```python
from build123d import *

# Parameters (mm, degrees)
SKETCH1_R           = 16.5
BOSS_EXTRUDE1_DEPTH = 0.44
SKETCH2_R           = 0.85
SKETCH2_W           = 7
SKETCH2_H           = 1.75
CUT_EXTRUDE1_DEPTH  = 0.44


with BuildPart() as part:
    # Sketch1 → Boss-Extrude1 (new body)
    with BuildSketch(Plane(origin=(0, 0, 0), x_dir=(1, 0, 0), z_dir=(0, 1, 0))):
        Circle(SKETCH1_R)
    extrude(amount=BOSS_EXTRUDE1_DEPTH)

    # Sketch2 → Cut-Extrude1 (cut)
    with BuildSketch(Plane(origin=(0, 0.44, 0), x_dir=(1, 0, 0), z_dir=(0, 1, 0))):
        Circle(SKETCH2_R)
        with Locations((6.95, 0)):
            Rectangle(SKETCH2_W, SKETCH2_H)
    extrude(amount=-CUT_EXTRUDE1_DEPTH, mode=Mode.SUBTRACT)


solid = part.part
```
Source: CAD feature listing. Evaluate the final solid. Frame: model axes, mm. Coordinates: 2 decimals unless noted, no trailing zeros. Write each loop counter-clockwise with the first axis right and the second up, starting at its lowest first coordinate (ties: lowest second). Pieces come first, ordered by that corner, then holes. Notation, with made-up numbers: (1.5, 0) -> (37.5, 0) arc R26 cw to (37.5, 17) -> close; hole circle Ø6 at (-11.75, -4.5). An arc over 180 degrees is marked (long way). Return JSON: item names as keys, results as strings. Group by question number.
1) Section query A-A, the plane z = 0. Return loops of the section in (x, y), plus the area to 3 significant figures.
2) Mould query, pull axis X, two halves, no side actions, for faces 1 (the face through (15.24, 0.22, 6.32)), 2 (the face through (0, 0.44, 3)), 3 (the face through (-0.18, 0.22, 0.83)). Classes: +X half, -X half, draft (parallel to the pull), parting line (faces both ways), or undercut.
3) Section query C-C, the plane y = 0.35. Return loops of the section in (x, z) (3 decimals), plus the area to 3 significant figures.
4) Section query B-B, the plane x = 0. Return loops of the section in (y, z), plus the area to 3 significant figures.
5) Ray query, line 1 along X through (y, z) = (0.25, 0); line 2 along Z through (x, y) = (0, 0.1); line 3 along X through (y, z) = (0.3, 6). Return the intervals inside material, ascending.
6) Section query D-D, the plane x = 14.5. Return loops of the section in (y, z), plus the area to 3 significant figures.
From the geometry:
{
 "1": {"outline": "(-16.5, 0) -> (-0.85, 0) -> (-0.85, 0.44) -> (-16.5, 0.44) -> close; (0.85, 0) -> (3.45, 0) -> (3.45, 0.44) -> (0.85, 0.44) -> close; (10.45, 0) -> (16.5, 0) -> (16.5, 0.44) -> (10.45, 0.44) -> close", "area": "10.7 mm²"},
 "2": {"face 1": "parting line", "face 2": "draft", "face 3": "undercut"},
 "3": {"outline": "circle Ø33 at (0, 0); hole circle Ø1.7 at (0, 0); hole (3.45, -0.875) -> (10.45, -0.875) -> (10.45, 0.875) -> (3.45, 0.875) -> close", "area": "841 mm²"},
 "4": {"outline": "(0, -16.5) -> (0.44, -16.5) -> (0.44, -0.85) -> (0, -0.85) -> close; (0, 0.85) -> (0.44, 0.85) -> (0.44, 16.5) -> (0, 16.5) -> close", "area": "13.8 mm²"},
 "5": {"line 1": "-16.5 to -0.85, 0.85 to 3.45, 10.45 to 16.5", "line 2": "-16.5 to -0.85, 0.85 to 16.5", "line 3": "-15.37 to 15.37"},
 "6": {"outline": "(0, -7.87) -> (0.44, -7.87) -> (0.44, 7.87) -> (0, 7.87) -> close", "area": "6.93 mm²"}
}
